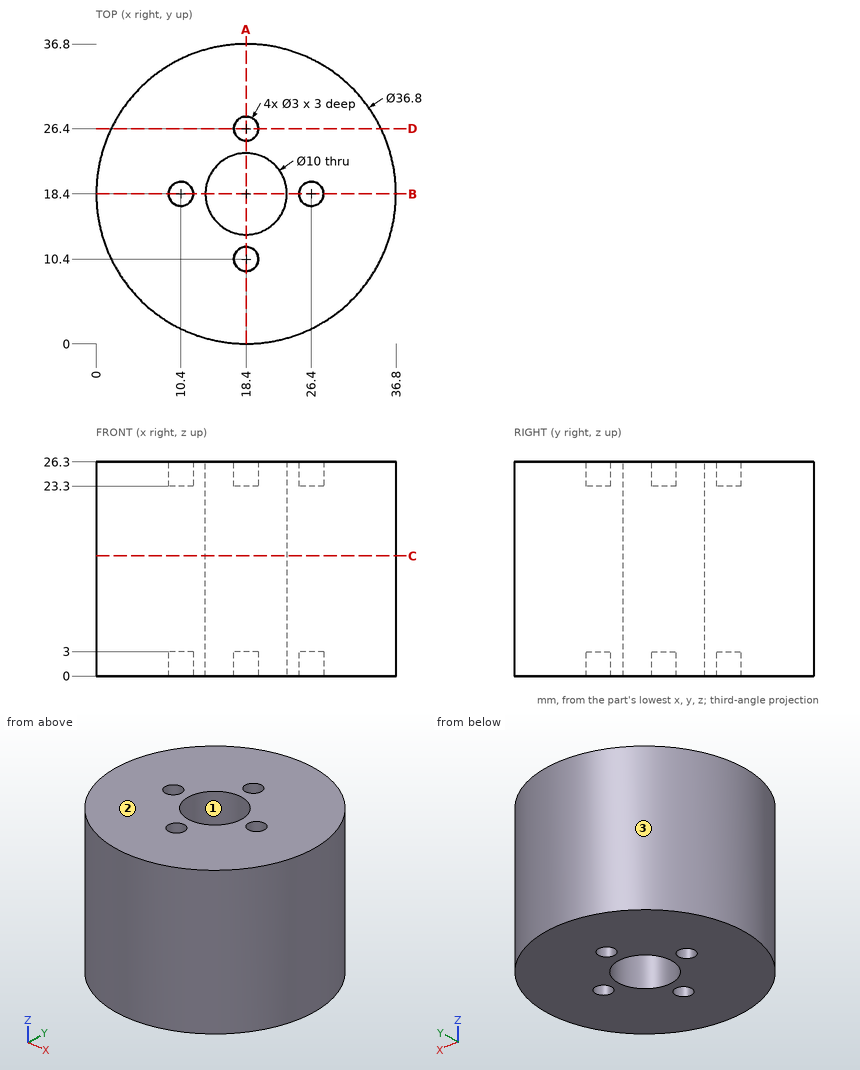
Answer from the drawing. Dimensions are ordinates in mm from the lowest x, y and z of the part. Coordinates: 2 decimals unless noted, no trailing zeros. Write each loop counter-clockwise with the first axis right and the second up, starting at its lowest first coordinate (ties: lowest second). Pieces come first, ordered by that corner, then holes. Notation, with made-up numbers: (53, 89.25) - (60, 89.25) arc R19 ccw to (60, 113.25) - close; hole circle Ø3 at (15, 47.5). An arc over 180 degrees is marked (long way). One line per question, with ' | ' between items.
Q1. Determine the mould class of the marked faces 1, 2 and 3 for opening direction Y: +Y half, -Y half, draft (parallel to the pull), parting line (faces both ways), or undercut.
Result set:
face 1: undercut | face 2: draft | face 3: parting line
Q2. Find section D-D, the plane y = 26.4. Write down the section's boundary in (x, z).
Result set:
outline: (1.83, 0) - (16.9, 0) - (16.9, 3) - (19.9, 3) - (19.9, 0) - (34.97, 0) - (34.97, 26.3) - (19.9, 26.3) - (19.9, 23.3) - (16.9, 23.3) - (16.9, 26.3) - (1.83, 26.3) - close
Q3. Each of these flat-tipped pins is pushed along its axis until it touches: P1, Ø1.8, axis at x = 26.4, y = 18.4, coming from the -Z side; P2, Ø9, axis at x = 18.4, y = 18.4, coming from the +Z side; P3, Ø2.5, axis at x = 18.4, y = 10.4, coming from the +Z side; P4, Ø3, axis at x = 24, z = 18, coming from the +Y side. Where does it stop, or does it pass through?
Result set:
P1: z = 3 | P2: through | P3: z = 23.3 | P4: y = 36.34
Q4. Find section A-A, the plane x = 18.4. Write down the section's boundary in (y, z).
Result set:
outline: (0, 0) - (8.9, 0) - (8.9, 3) - (11.9, 3) - (11.9, 0) - (13.4, 0) - (13.4, 26.3) - (11.9, 26.3) - (11.9, 23.3) - (8.9, 23.3) - (8.9, 26.3) - (0, 26.3) - close; (23.4, 0) - (24.9, 0) - (24.9, 3) - (27.9, 3) - (27.9, 0) - (36.8, 0) - (36.8, 26.3) - (27.9, 26.3) - (27.9, 23.3) - (24.9, 23.3) - (24.9, 26.3) - (23.4, 26.3) - close
Q5. Find section C-C, the plane z = 14.75. Write down the section's boundary in (x, y), plus the area to 3 significant figures.
Result set:
outline: circle Ø36.8 at (18.4, 18.4); hole circle Ø10 at (18.4, 18.4) | area: 985 mm^2
Q6. Consider L1, parallel to Y at x = 18.4, z = 24.75; L2, parallel to X at y = 16.5, z = 21.25; L3, parallel to Y at x = 17.5, z = 12. Determine where each line is inside the solid, lowest interval first. Write a range as [from, to].
Result set:
L1: [0, 8.9], [11.9, 13.4], [23.4, 24.9], [27.9, 36.8] | L2: [0.1, 13.78], [23.02, 36.7] | L3: [0.02, 13.48], [23.32, 36.78]
